Verification items for the finished model (mm, model axes). Round coordinates to 2 decimals unless told otherwise and drop trailing zeros. Write each loop counter-clockwise with the first axis right and the second up, starting at its lowest first coordinate (ties: lowest second). Pieces come first, ordered by that corner, then holes. Notation, with made-up numbers: (65, -29) -> (82, -29) arc R32 cw to (82, 6) -> close; hole circle Ø4 at (-35.5, 1.5). An arc over 180 degrees is marked (long way). Answer as a JSON object with one key per item and string values. Group by question number.
(1) Gauge pin test, flat end, axial feed: pin 1 Ø1.8 at (x, y) = (25.75, -11.69) entering from +Z. Record the tip position at first contact, or that the pin passes through.
(2) Scan lines: L1, parallel to Y at x = -13, z = 0.45; L2, parallel to Y at x = 25.75, z = 2; L3, parallel to Y at x = 39.25, z = 1.6. Record each from-to range of solid material in increasing order. Write a range as from..to.
(3) Sectioned sample at C-C on y = -6.5. Record the cut outline in (x, z).
(4) Sectioned sample at B-B on x = 4. Record the cut outline in (y, z).
(5) Sectioned sample at A-A on y = 0. Record the cut outline in (x, z).
(6) Sectioned sample at D-D on x = 19. Record the cut outline in (y, z), and give its area (3 significant figures).
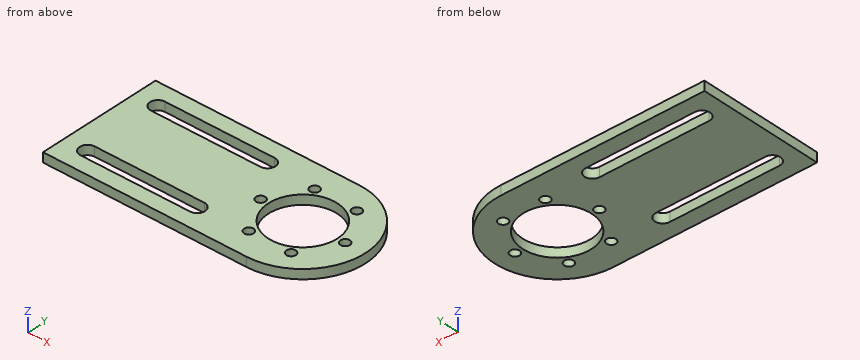
```python
from build123d import *

# Parameters (mm, degrees)
SKETCH1_R           = 11
BOSS_EXTRUDE1_DEPTH = 3
SKETCH2_R           = 1.5
CUT_EXTRUDE1_DEPTH  = 3
CIRPATTERN1_COUNT   = 6


with BuildPart() as part:
    # Sketch1 → Boss-Extrude1 (new body)
    with BuildSketch(Plane.XY):
        with BuildLine():
            Line((32.5, 20), (-32.5, 20))
            Line((-32.5, 20), (-32.5, -20))
            Line((-32.5, -20), (32.5, -20))
            ThreePointArc((32.5, -20), (52.5, 0), (32.5, 20))
        make_face()
        with Locations((32.5, 0)):
            Circle(SKETCH1_R, mode=Mode.SUBTRACT)
        with BuildLine():
            Line((-25, 15), (10, 15))
            ThreePointArc((10, 15), (12.5, 12.5), (10, 10))
            Line((10, 10), (-25, 10))
            ThreePointArc((-25, 10), (-27.5, 12.5), (-25, 15))
        make_face(mode=Mode.SUBTRACT)
        with BuildLine():
            Line((-25, -10), (10, -10))
            ThreePointArc((10, -10), (12.5, -12.5), (10, -15))
            Line((10, -15), (-25, -15))
            ThreePointArc((-25, -15), (-27.5, -12.5), (-25, -10))
        make_face(mode=Mode.SUBTRACT)
    extrude(amount=BOSS_EXTRUDE1_DEPTH)

    # Sketch2 → Cut-Extrude1 (cut)
    with BuildSketch(Plane.XY.offset(3)):
        with Locations((46, 0)):
            Circle(SKETCH2_R)
    cut_extrude1 = extrude(amount=-CUT_EXTRUDE1_DEPTH, mode=Mode.SUBTRACT)

    # CirPattern1: Cut-Extrude1 ×6 about axis
    cirpattern1_axis = Axis((32.5, 0, 0), (0, 0, 1))
    for i in range(1, CIRPATTERN1_COUNT):
        add(cut_extrude1.rotate(cirpattern1_axis, i * 360 / CIRPATTERN1_COUNT), mode=Mode.SUBTRACT)


solid = part.part
```
Computed values:
{
 "1": {"pin 1": "through"},
 "2": {"L1": "-20..-15, -10..10, 15..20", "L2": "-20..-13.19, -10.19..-8.69, 8.69..10.19, 13.19..20", "L3": "-18.83..-13.19, -10.19..-8.69, 8.69..10.19, 13.19..18.83"},
 "3": {"outline": "(-32.5, 0) -> (23.63, 0) -> (23.63, 3) -> (-32.5, 3) -> close; (41.37, 0) -> (51.41, 0) -> (51.41, 3) -> (41.37, 3) -> close"},
 "4": {"outline": "(-20, 0) -> (-15, 0) -> (-15, 3) -> (-20, 3) -> close; (-10, 0) -> (10, 0) -> (10, 3) -> (-10, 3) -> close; (15, 0) -> (20, 0) -> (20, 3) -> (15, 3) -> close"},
 "5": {"outline": "(-32.5, 0) -> (17.5, 0) -> (17.5, 3) -> (-32.5, 3) -> close; (20.5, 0) -> (21.5, 0) -> (21.5, 3) -> (20.5, 3) -> close; (43.5, 0) -> (44.5, 0) -> (44.5, 3) -> (43.5, 3) -> close; (47.5, 0) -> (52.5, 0) -> (52.5, 3) -> (47.5, 3) -> close"},
 "6": {"outline": "(-20, 0) -> (-1.5, 0) -> (-1.5, 3) -> (-20, 3) -> close; (1.5, 0) -> (20, 0) -> (20, 3) -> (1.5, 3) -> close", "area": "111 mm2"}
}
